Autodesk Inventor part; units mm, degrees
ref_plane "YZ Plane" through (0, 0, 0) normal (1, 0, 0) x (0, 1, 0)
ref_plane "XZ Plane" through (0, 0, 0) normal (0, 1, 0) x (-1, 0, 0)
ref_plane "XY Plane" through (0, 0, 0) normal (0, 0, 1) x (1, 0, 0)
sketch "Sketch1" plane through (0, 0, 0) normal (0, 0, 1) x (1, 0, 0)
  line L0 (0, 0) -> (0, 49.7586)
  line L1 (0, 49.7586) -> (187.6422, 59.5597)
  line L2 (187.6422, 59.5597) -> (0, 0)
  dimension "d0" = 49.7586
  dimension "d40" = 92.99
  dimension "d41" = 72.39
extrude "Extrusion1" add sketch "Sketch1" along normal blind 3.175
sketch "Sketch3" plane through (0, 0, 3.175) normal (0, 0, 1) x (1, 0, 0)
  line L0 (0, 49.7586) -> (0, 0)
  line L1 (0, 27.1018) -> (-3.175, 27.1018)
  line L2 (-3.175, 27.1018) -> (-3.175, 19.4818)
  line L3 (-3.175, 19.4818) -> (0, 19.4818)
  line L4 (0, 27.1018) -> (0, 19.4818)
  point P0 (0, 23.2918)
  dimension "d9" = 7.62
  dimension "d11" = 3.175
  dimension "d43" = 26.4668
  dimension "d44" = 3.81
extrude "Extrusion3" add sketch "Sketch3" against normal blind 3.175
sketch "Sketch5" plane through (0, 0, 3.175) normal (0, 0, 1) x (1, 0, 0)
  line L0 (187.6422, 59.5597) -> (0, 49.7586)
  line L1 (0, 0) -> (187.6422, 59.5597)
  line L2 (92.766, 54.604) -> (92.9316, 51.4333)
  line L3 (92.9316, 51.4333) -> (100.5412, 51.8308)
  line L4 (100.5412, 51.8308) -> (100.3756, 55.0015)
  line L5 (92.766, 54.604) -> (100.3756, 55.0015)
  line L6 (100.2023, 31.8053) -> (99.2417, 34.8315)
  line L7 (99.2417, 34.8315) -> (91.9788, 32.5262)
  line L8 (91.9788, 32.5262) -> (92.9393, 29.5)
  line L9 (92.9393, 29.5) -> (100.2023, 31.8053)
  point P0 (96.5708, 54.8028)
  point P1 (96.5708, 30.6526)
  dimension "d32" = 7.62
  dimension "d34" = 3.175
  dimension "d35" = 3.175
  dimension "d36" = 7.62
  dimension "d45" = 96.5708
  dimension "d46" = 96.5708
  dimension "d47" = 3.81
  dimension "d48" = 3.81
extrude "Extrusion5" cut sketch "Sketch5" against normal blind 25.4
sketch "Sketch6" plane through (0, 0, 3.175) normal (0, 0, 1) x (1, 0, 0)
  line L0 (0, 0) -> (0, 19.4818)
  line L1 (0, 19.4818) -> (0, 0)
  line L2 (0, 19.4818) -> (-3.175, 19.4818)
  line L3 (-3.175, 19.4818) -> (0, 19.4818)
  line L4 (-3.175, 19.4818) -> (-3.175, 27.1018)
  line L5 (-3.175, 27.1018) -> (-3.175, 19.4818)
  line L6 (-3.175, 27.1018) -> (0, 27.1018)
  line L7 (0, 27.1018) -> (-3.175, 27.1018)
  line L8 (0, 27.1018) -> (0, 49.7586)
  line L9 (0, 49.7586) -> (0, 27.1018)
  line L10 (0, 49.7586) -> (92.766, 54.604)
  line L11 (92.766, 54.604) -> (0, 49.7586)
  line L12 (92.766, 54.604) -> (92.9316, 51.4333)
  line L13 (92.9316, 51.4333) -> (100.5412, 51.8308)
  line L14 (100.5412, 51.8308) -> (92.9316, 51.4333)
  line L15 (100.5412, 51.8308) -> (100.3756, 55.0015)
  line L16 (100.3756, 55.0015) -> (100.5412, 51.8308)
  line L17 (100.3756, 55.0015) -> (187.6422, 59.5597)
  line L18 (100.3756, 55.0015) -> (187.6422, 59.5597)
  line L19 (187.6422, 59.5597) -> (100.2023, 31.8053)
  line L20 (100.2023, 31.8053) -> (187.6422, 59.5597)
  line L21 (100.2023, 31.8053) -> (99.2417, 34.8315)
  line L22 (99.2417, 34.8315) -> (91.9788, 32.5262)
  line L23 (91.9788, 32.5262) -> (92.9393, 29.5)
  line L24 (91.9788, 32.5262) -> (92.9393, 29.5)
  line L25 (92.9393, 29.5) -> (0, 0)
properties part number "Star Side" material "Wood (Birch)"
Could you check a few things on this model? Use its own coordinates, in mm. A direction names the side the tool comes from. Coordinates: 2 decimals unless noted, no trailing zeros. Order: outer loops, then holes, each group sorted by start corner. A loop starts at its lowest first (then second) coordinate and runs counter-clockwise, first axis right, second up. Notation, with made-up numbers: M -39,40 L -3,40 A22 cw -3,55 Z; hole C -6,26.5 d5. An arc over 180 degrees is marked long. Use a Markdown table: item, result. Add a question column.
Q1. I want a section at A-A on z = 2. List the corners of the cut face in (x, y) for me (1 decimal).
Q2. I want a section at B-B on x = 50. List the corners of the cut face in (y, z) for me (3 decimals).
Q3. I want a section at C-C on y = 41.5. List the corners of the cut face in (x, z) for me (3 decimals).
Q4. We'd pull the mould along Y, two halves only. Please class faces 5 (the flat face through (144.534, 45.877, 1.565)), 6 (the flat face through (92.452, 31.034, 1.61)), 7 (the flat face through (-3.175, 23, 2)): pulls with the +Y half, pulls with the -Y half, needs draft (parallel to the pull), parting line crosses it, or undercut.
Q5. If I drill on L1, parallel to Y at x = 109.5, z = 1.9; L2, parallel to Y at x = 157, z = 0.3, over which ranges is the centre line in solid material (lowest first)?
Q6. I'm going to push flat-ended pins straight in: pin 1 (1 mm diameter, centred on y = 10, z = 1, fed in from -X); pin 2 (1.6 mm diameter, centred on x = -1.5, z = 2.5, fed in from -Y). Where does each tip first touch, or does it pass through?
Q7. Which directions (+Z, -Z, +X, -X, +Y, -Y) give clear straight access to the entire face, cutting with the end or side of a thin tool? Please do faces 1 (the flat face through (100.46, 53.39, 1.61)), 2 (the flat face through (-2, 27.102, 2)), 3 (the flat face through (92.848, 53.041, 1.61)), 4 (the flat face through (0, 10, 2)).
Checked values:
| question | item | result |
|---|---|---|
| 1 | outline | M -3.2,19.5 L 0,19.5 L 0,0 L 92.9,29.5 L 92,32.5 L 99.2,34.8 L 100.2,31.8 L 187.6,59.6 L 100.4,55 L 100.5,51.8 L 92.9,51.4 L 92.8,54.6 L 0,49.8 L 0,27.1 L -3.2,27.1 Z |
| 2 | outline | M 15.871,0 L 52.37,0 L 52.37,3.175 L 15.871,3.175 Z |
| 3 | outline | M 0,0 L 130.745,0 L 130.745,3.175 L 0,3.175 Z |
| 4 | face 5 | pulls with the -Y half |
| 4 | face 6 | undercut |
| 4 | face 7 | needs draft |
| 5 | L1 | 34.76 to 55.48 |
| 5 | L2 | 49.83 to 57.96 |
| 6 | pin 1 | x = 0 |
| 6 | pin 2 | y = 19.48 |
| 7 | face 1 | +Z, -Z |
| 7 | face 2 | +Z, -Z, -X, +Y |
| 7 | face 3 | +Z, -Z, +Y |
| 7 | face 4 | +Z, -Z, -X, -Y |
